from build123d import *

# Parameters (mm, degrees)
SKETCH1_R           = 254
BOSS_EXTRUDE1_DEPTH = 1270
SKETCH2_R           = 304.8
BOSS_EXTRUDE2_DEPTH = 381
CUT_EXTRUDE1_DEPTH  = 304.8
SKETCH4_W           = 152.4
SKETCH4_H           = 635
CUT_EXTRUDE2_DEPTH  = 101.6


with BuildPart() as part:
    # Sketch1 → Boss-Extrude1 (new body)
    with BuildSketch(Plane(origin=(0, 0, 0), x_dir=(1, 0, 0), z_dir=(0, 1, 0))):
        Circle(SKETCH1_R)
    extrude(amount=-BOSS_EXTRUDE1_DEPTH)

    # Sketch2 → Boss-Extrude2 (add)
    with BuildSketch(Plane(origin=(0, 0, 0), x_dir=(1, 0, 0), z_dir=(0, 1, 0))):
        Circle(SKETCH2_R)
    extrude(amount=BOSS_EXTRUDE2_DEPTH)

    # Sketch3 → Cut-Extrude1 (cut)
    with BuildSketch(Plane(origin=(0, 381, 0), x_dir=(1, 0, 0), z_dir=(0, 1, 0))):
        Polygon((-127.035376657, 220.031726729), (127.035376657, 220.031726729), (254.070753314, 0), (127.035376657, -220.031726729), (-127.035376657, -220.031726729), (-254.070753314, 0), align=None)
    extrude(amount=-CUT_EXTRUDE1_DEPTH, mode=Mode.SUBTRACT)

    # Sketch4 → Cut-Extrude2 (cut)
    with BuildSketch(Plane.XY.offset(-254)):
        with Locations((0, -508)):
            Rectangle(SKETCH4_W, SKETCH4_H)
    extrude(amount=CUT_EXTRUDE2_DEPTH, mode=Mode.SUBTRACT)


solid = part.part
Read the model definition and answer for the solid it produces. Units are mm, in the model's axes. A direction names the side the tool comes from. Round coordinates to 2 decimals unless told otherwise and drop trailing zeros. Write each loop counter-clockwise with the first axis right and the second up, starting at its lowest first coordinate (ties: lowest second). Pieces come first, ordered by that corner, then holes.
Q1. The mould has two halves that part along Z. Classify faces 1 (the face through (189.66, 230.73, -111.56)), 2 (the face through (-4, -1270, -4)), 3 (the face through (-189.66, 230.73, 111.56)), 4 (the face through (-1, -504, -152.4)): released by +Z, released by -Z, zero draft, split by the parting line, or undercut.
Values:
face 1: undercut
face 2: zero draft
face 3: undercut
face 4: released by -Z
Q2. Straight lines are drawn through the part: line 1 (Y direction, x = -10, z = -208); line 2 (Y direction, x = -49.5, z = -39.5); line 3 (Y direction, x = -216, z = 166). For each, find the intervals that lie inside material, in ascending order.
Values:
line 1: y = -1270 to -825.5, -190.5 to 76.2
line 2: y = -1270 to 76.2
line 3: y = 0 to 381
Q3. A tool of negligible diameter and unlimited length cuts with its end or side. For faces 5 (the face through (-2, 231, -220.032)), 6 (the face through (-241.879, 187.833, 185.466)), 7 (the face through (-182, 381, 134)), 8 (the face through (-1, -190.5, -204)), 9 (the face through (-55.06, -626.11, 247.96)), from which of +Z, -Z, +X, -X, +Y, -Y can it reach the whole face along a straight path? Write none if from no direction.
Values:
face 5: +Y
face 6: +Y, -Y
face 7: +Z, -Z, +X, -X, +Y
face 8: -Z
face 9: -Y
Q4. Find section A-A on y = 246.5. Determine the outline of the cut face in (x, z), and give its area (3 significant figures).
Values:
outline: circle Ø609.6 at (0, 0); hole (-254.07, 0) - (-127.04, -220.03) - (127.04, -220.03) - (254.07, 0) - (127.04, 220.03) - (-127.04, 220.03) - close
area: 124,000 mm2
Q5. Flat-ended cylindrical pins translate along their axes: P1, Ø8, axis at y = -258, z = -164.5, coming from the +X side; P2, Ø4, axis at x = 143.5, y = -815, coming from the -Z side; P3, Ø3, axis at y = -746.5, z = -203.5, coming from the -X side. Find the tip coordinate at first contact, or state that the pin passes through.
Values:
P1: stops at x = 196.86
P2: stops at z = -210.94
P3: stops at x = -153.99
Q6. Find section C-C on z = -201.5. Determine the outline of the cut face in (x, y), and give its area (3 significant figures).
Values:
outline: (-228.69, 0) - (-154.64, 0) - (-154.64, -1270) - (154.64, -1270) - (154.64, 0) - (228.69, 0) - (228.69, 381) - (137.73, 381) - (137.73, 76.2) - (-137.73, 76.2) - (-137.73, 381) - (-228.69, 381) - close; hole (-76.2, -825.5) - (76.2, -825.5) - (76.2, -190.5) - (-76.2, -190.5) - close
area: 386,000 mm2
Q7. Find section B-B on x = 0. Determine the outline of the cut face in (y, z).
Values:
outline: (-1270, -254) - (-825.5, -254) - (-825.5, -152.4) - (-190.5, -152.4) - (-190.5, -254) - (0, -254) - (0, -304.8) - (381, -304.8) - (381, -220.03) - (76.2, -220.03) - (76.2, 220.03) - (381, 220.03) - (381, 304.8) - (0, 304.8) - (0, 254) - (-1270, 254) - close
Q8. Find section D-D on y = -653. Determine the outline of the cut face in (x, z).
Values:
outline: (-76.2, -242.3) - (-76.2, -152.4) - (76.2, -152.4) - (76.2, -242.3) arc R254 ccw (long way) to start
